Verification items for the finished model (mm, model axes). A direction names the side the tool comes from. Round coordinates to 2 decimals unless told otherwise and drop trailing zeros. Order: outer loops, then holes, each group sorted by start corner. A loop starts at its lowest first (then second) coordinate and runs counter-clockwise, first axis right, second up. Notation, with made-up numbers: (38, 36) -> (84, 36) arc R17 ccw to (84, 57) -> close; hole circle Ø5 at (-3.5, 46.5). An arc over 180 degrees is marked (long way). Write item = value, one per line. Start each with the question number.
from build123d import *

# Parameters (mm, degrees)
ESQUISSE1_W             = 32
ESQUISSE1_H             = 80
ESQUISSE1_R             = 1.25
BOSS_EXTRU_2_DEPTH      = 8
ENL_V_MAT_EXTRU_1_DEPTH = 5


with BuildPart() as part:
    # Esquisse1 → Boss.-Extru.2 (new body)
    with BuildSketch(Plane.XY):
        with Locations((16, 40)):
            Rectangle(ESQUISSE1_W, ESQUISSE1_H)
        with Locations((2, 78.5)):
            Circle(ESQUISSE1_R, mode=Mode.SUBTRACT)
        with Locations((30, 78.5)):
            Circle(ESQUISSE1_R, mode=Mode.SUBTRACT)
        with Locations((16, 1.5)):
            Circle(ESQUISSE1_R, mode=Mode.SUBTRACT)
    extrude(amount=BOSS_EXTRU_2_DEPTH)

    # Esquisse2 → Enlèv. mat.-Extru.1 (cut)
    with BuildSketch(Plane.XY.offset(8)):
        with BuildLine():
            Line((24, 68), (29, 68))
            ThreePointArc((29, 68), (29.707106781, 67.707106781), (30, 67))
            Line((30, 67), (30, 13))
            ThreePointArc((30, 13), (29.707106781, 12.292893219), (29, 12))
            Line((29, 12), (24, 12))
            ThreePointArc((24, 12), (23.292893219, 12.292893219), (23, 13))
            Line((23, 13), (23, 67))
            ThreePointArc((23, 67), (23.292893219, 67.707106781), (24, 68))
        make_face()
        with BuildLine():
            Line((3, 72), (13, 72))
            ThreePointArc((13, 72), (13.707106781, 71.707106781), (14, 71))
            Line((14, 71), (14, 13))
            ThreePointArc((14, 13), (13.707106781, 12.292893219), (13, 12))
            Line((13, 12), (3, 12))
            ThreePointArc((3, 12), (2.292893219, 12.292893219), (2, 13))
            Line((2, 13), (2, 71))
            ThreePointArc((2, 71), (2.292893219, 71.707106781), (3, 72))
        make_face()
    extrude(amount=-ENL_V_MAT_EXTRU_1_DEPTH, mode=Mode.SUBTRACT)


solid = part.part
(1) Scan lines: line 1 along X through (y, z) = (47, 7.75); line 2 along X through (y, z) = (78.5, 6.25); line 3 along Y through (x, z) = (16, 2). Record each from-to range of solid material in increasing order. Write a range as from..to.
(2) Cross-section at B-B (z = 4). Enter the section's corners in (x, y), and give its area (3 significant figures).
(3) Cross-section at A-A (y = 78.5). Enter the section's corners in (x, z).
(4) Cross-section at C-C (x = 16). Enter the section's corners in (y, z).
(5) Set-up check for faces 5 (the flat face through (26, 68, 6)), 6 (the cylindrical face through (15.73, 0.28, 3.94)): record each of +Z, -Z, +X, -X, +Y, -Y from which the full face is reachable in a straight line by a thin tool's end or side.
(6) Draft check along Y on faces 1 (the flat face through (16, 41, 0)), 2 (the cylindrical face through (1.84, 79.74, 3.94)), 3 (the flat face through (16, 0, 4)), 4 (the cylindrical face through (29.84, 79.74, 3.94)). Enter one of: +Y half, -Y half, draft (parallel to the pull), parting line (faces both ways), or undercut.
(7) Depth check by flat-ended pin: pin 1 (5.5 mm diameter, centred on x = 26.5, y = 43, fed in from +Z). Enter the tip coordinate at first touch or a pass-through.
(8) Cross-section at D-D (x = 27). Enter the section's corners in (y, z).
Outcome:
q1.line_1 = 0..2, 14..23, 30..32
q1.line_2 = 0..0.75, 3.25..28.75, 31.25..32
q1.line_3 = 0..0.25, 2.75..80
q2.outline = (0, 0) -> (32, 0) -> (32, 80) -> (0, 80) -> close; hole circle Ø2.5 at (2, 78.5); hole (2, 13) arc R1 ccw to (3, 12) -> (13, 12) arc R1 ccw to (14, 13) -> (14, 71) arc R1 ccw to (13, 72) -> (3, 72) arc R1 ccw to (2, 71) -> close; hole circle Ø2.5 at (16, 1.5); hole (23, 13) arc R1 ccw to (24, 12) -> (29, 12) arc R1 ccw to (30, 13) -> (30, 67) arc R1 ccw to (29, 68) -> (24, 68) arc R1 ccw to (23, 67) -> close; hole circle Ø2.5 at (30, 78.5)
q2.area = 1,430 mm^2
q3.outline = (0, 0) -> (0.75, 0) -> (0.75, 8) -> (0, 8) -> close; (3.25, 0) -> (28.75, 0) -> (28.75, 8) -> (3.25, 8) -> close; (31.25, 0) -> (32, 0) -> (32, 8) -> (31.25, 8) -> close
q4.outline = (0, 0) -> (0.25, 0) -> (0.25, 8) -> (0, 8) -> close; (2.75, 0) -> (80, 0) -> (80, 8) -> (2.75, 8) -> close
q5.face_5 = +Z
q5.face_6 = +Z, -Z
q6.face_1 = draft
q6.face_2 = undercut
q6.face_3 = -Y half
q6.face_4 = undercut
q7.pin_1 = 3
q8.outline = (0, 0) -> (80, 0) -> (80, 8) -> (68, 8) -> (68, 3) -> (12, 3) -> (12, 8) -> (0, 8) -> close
